```python
from build123d import *

# Parameters (mm, degrees)
SKETCH1_R           = 3.175
EXTRUDE1_DEPTH      = 22.225
SKETCH2_R           = 4.826
EXTRUDE2_DEPTH      = 2.54
CHAMFER1_SIZE       = 0.508
SKETCH3_R           = 1.190625
EXTRUDE3_DEPTH      = 5.826
EXTRUDE3_DEPTH_BACK = 5.826
CHAMFER2_SIZE       = 0.3175


with BuildPart() as part:
    # Sketch1 → Extrude1 (new body, symmetric)
    with BuildSketch(Plane.XY):
        Circle(SKETCH1_R)
    extrude(amount=EXTRUDE1_DEPTH, both=True)

    # Sketch2 → Extrude2 (add)
    with BuildSketch(Plane.XY.offset(22.225)):
        Circle(SKETCH2_R)
    extrude(amount=EXTRUDE2_DEPTH)

    # Chamfer1
    chamfer1_edges = [part.edges().sort_by_distance(p)[0] for p in [
        (-4.826, 0, 24.765),
    ]]
    chamfer(chamfer1_edges, length=CHAMFER1_SIZE)

    # Sketch3 → Extrude3 (cut, two sides)
    with BuildSketch(Plane(origin=(0, 0, 0), x_dir=(0, 0, -1), z_dir=(1, 0, 0))) as extrude3_sk:
        with Locations((18.653125, 0)):
            Circle(SKETCH3_R)
    extrude(amount=EXTRUDE3_DEPTH, mode=Mode.SUBTRACT)
    extrude(extrude3_sk.sketch, amount=-EXTRUDE3_DEPTH_BACK, mode=Mode.SUBTRACT)

    # Chamfer2
    chamfer2_edges = [part.edges().sort_by_distance(p)[0] for p in [
        (-3.175, 0, -22.225),
    ]]
    chamfer(chamfer2_edges, length=CHAMFER2_SIZE)


solid = part.part
```
Geometry: final body of the model. Coordinates: model frame, mm. A direction names the side the tool comes from. Give positions to 0.01 mm unless a question says otherwise; leave off trailing zeros. Loops run counter-clockwise (first coordinate to the right, second up) from the corner with the lowest first, then second, coordinate; pieces in that order, holes last. Notation, with made-up numbers: (8.25, 49.25) -> (53.25, 49.25) arc R17 ccw to (53.25, 57.25) -> close; hole circle Ø10 at (-18, 31.25). An arc over 180 degrees is marked (long way). Use one line per item in the form item = value.
Item 1: Section query A-A on z = -0.5. Output: boundary loops of the cut face in (x, y) (3 decimals), and give its area (3 significant figures).
A:
outline = circle Ø6.35 at (0, 0)
area = 31.7 mm^2
Item 2: Pin query (flat end, axial travel): P1, Ø2, axis at x = 3, z = 19.5, coming from the +Y side; P2, Ø2.5, axis at y = 0, z = -18.65, coming from the +X side (3 decimals); P3, Ø1, axis at x = 2.5, z = 4.5, coming from the -Y side. Return the tip coordinate at first contact, or that it passes through.
A:
P1 = 2.47
P2 = 3.175
P3 = -2.47
Item 3: Line query: probe 1 along Z at (x, y) = (-2.15, 0) (1 decimal); probe 2 along Y at (x, z) = (-0.25, 22); probe 3 along X at (y, z) = (1.5, -15). Output: solid intervals per line, ascending.
A:
probe_1 = -22.2 to -19.8, -17.5 to 24.8
probe_2 = -3.17 to 3.17
probe_3 = -2.8 to 2.8
Item 4: Access query for faces 1 (the face through (-0.69, -3.1, 0.47)), 2 (the face through (0, 0, 24.765)). Directions: +Z, -Z, +X, -X, +Y, -Y. A direction counts if a zero-diameter tool reaches every point of the face in a straight line with its end or side. Return the directions, or none.
A:
face_1 = -Z
face_2 = +Z, +X, -X, +Y, -Y
